from build123d import *

# Parameters (mm, degrees)
SKETCH1_R           = 6.75
BOSS_EXTRUDE1_DEPTH = 6
SKETCH2_R           = 3.5
BOSS_EXTRUDE2_DEPTH = 43


with BuildPart() as part:
    # Sketch1 → Boss-Extrude1 (new body)
    with BuildSketch(Plane(origin=(0, 0, 0), x_dir=(1, 0, 0), z_dir=(0, 1, 0))):
        with BuildLine():
            Line((-35, 10), (35, 10))
            ThreePointArc((35, 10), (45, 0), (35, -10))
            Line((35, -10), (-35, -10))
            ThreePointArc((-35, -10), (-45, 0), (-35, 10))
        make_face()
        with Locations(Location((0, 0, 0), (0, 0, 270))):
            Circle(SKETCH1_R, mode=Mode.SUBTRACT)
        with Locations(Location((35, 0, 0), (0, 0, 270))):
            Circle(SKETCH1_R, mode=Mode.SUBTRACT)
        with Locations(Location((-35, 0, 0), (0, 0, 270))):
            Circle(SKETCH1_R, mode=Mode.SUBTRACT)
    extrude(amount=BOSS_EXTRUDE1_DEPTH)

    # Sketch2 → Boss-Extrude2 (add)
    with BuildSketch(Plane(origin=(0, 6, 0), x_dir=(1, 0, 0), z_dir=(0, 1, 0))):
        with BuildLine():
            Line((-35, -10), (35, -10))
            ThreePointArc((35, -10), (45, 0), (35, 10))
            Line((35, 10), (-35, 10))
            ThreePointArc((-35, 10), (-45, 0), (-35, -10))
        make_face()
        with Locations(Location((-35, 0, 0), (0, 0, 270))):
            Circle(SKETCH2_R, mode=Mode.SUBTRACT)
        with Locations(Location((0, 0, 0), (0, 0, 270))):
            Circle(SKETCH2_R, mode=Mode.SUBTRACT)
        with Locations(Location((35, 0, 0), (0, 0, 270))):
            Circle(SKETCH2_R, mode=Mode.SUBTRACT)
    extrude(amount=BOSS_EXTRUDE2_DEPTH)


solid = part.part
Input: part model. Units: mm. Frame: model coordinates. A direction names the side the tool comes from. Give positions to 0.01 mm unless a question says otherwise; leave off trailing zeros. Write each loop counter-clockwise with the first axis right and the second up, starting at its lowest first coordinate (ties: lowest second). Pieces come first, ordered by that corner, then holes.
Q1. Pull-direction query (Z, two-part tool) for faces 1 (the face through (-1, 49, 4)), 2 (the face through (45, 24, 0)), 3 (the face through (38.47, 27.2, -0.46)), 4 (the face through (0, 24, -10)); classes: pulls with the +Z half, pulls with the -Z half, needs draft (parallel to the pull), parting line crosses it, or undercut.
Q2. First-contact query: P1, Ø9, axis at x = -35, z = 0, coming from the +Y side; P2, Ø8, axis at x = 35, z = 0, coming from the -Y side. Flat tips, straight axial feed; report the tip coordinate or a pass-through.
Q3. Section B-B, the plane x = 0. Output: boundary loops of the cut face in (y, z).
Q4. Section A-A, the plane z = 0. Output: boundary loops of the cut face in (x, y).
Q5. Set-up query: faces 5 (the face through (1, 0, -7)), 6 (the face through (-6.59, 2.96, -1.46)). Return all of +Z, -Z, +X, -X, +Y, -Y with unobstructed straight access to the full face (end or side cutting, diameter ignored); none if empty.
Q6. Section D-D, the plane z = 5.5. Output: boundary loops of the cut face in (x, y).
Q7. Section C-C, the plane y = 14. Output: boundary loops of the cut face in (x, z).
Q8. Material intervals for probe 1 along X at (y, z) = (3.2, 0); probe 2 along X at (y, z) = (36, -0.5); probe 3 along Z at (x, y) = (-33.5, 43), sorted ascending.
Filled in:
1. face 1: needs draft
1. face 2: parting line crosses it
1. face 3: undercut
1. face 4: pulls with the -Z half
2. P1: stops at y = 49
2. P2: stops at y = 6
3. outline: (0, -10) - (49, -10) - (49, -3.5) - (6, -3.5) - (6, -6.75) - (0, -6.75) - close; (0, 6.75) - (6, 6.75) - (6, 3.5) - (49, 3.5) - (49, 10) - (0, 10) - close
4. outline: (-45, 0) - (-41.75, 0) - (-41.75, 6) - (-38.5, 6) - (-38.5, 49) - (-45, 49) - close; (-31.5, 6) - (-28.25, 6) - (-28.25, 0) - (-6.75, 0) - (-6.75, 6) - (-3.5, 6) - (-3.5, 49) - (-31.5, 49) - close; (3.5, 6) - (6.75, 6) - (6.75, 0) - (28.25, 0) - (28.25, 6) - (31.5, 6) - (31.5, 49) - (3.5, 49) - close; (38.5, 6) - (41.75, 6) - (41.75, 0) - (45, 0) - (45, 49) - (38.5, 49) - close
5. face 5: +Z, -Z, +X, -X, -Y
5. face 6: -Y
6. outline: (-43.35, 0) - (-38.91, 0) - (-38.91, 6) - (-31.09, 6) - (-31.09, 0) - (-3.91, 0) - (-3.91, 6) - (3.91, 6) - (3.91, 0) - (31.09, 0) - (31.09, 6) - (38.91, 6) - (38.91, 0) - (43.35, 0) - (43.35, 49) - (-43.35, 49) - close
7. outline: (-35, -10) - (35, -10) arc R10 ccw to (35, 10) - (-35, 10) arc R10 ccw to start; hole circle Ø7 at (-35, 0); hole circle Ø7 at (0, 0); hole circle Ø7 at (35, 0)
8. probe 1: x = -45 to -41.75, -28.25 to -6.75, 6.75 to 28.25, 41.75 to 45
8. probe 2: x = -44.99 to -38.46, -31.54 to -3.46, 3.46 to 31.54, 38.46 to 44.99
8. probe 3: z = -10 to -3.16, 3.16 to 10
